```python
from build123d import *

# Parameters (mm, degrees)
SKETCH1_W           = 4.8
SKETCH1_H           = 4.8
BOSS_EXTRUDE1_DEPTH = 20
SKETCH2_W           = 5.2
SKETCH2_H           = 5.2
BOSS_EXTRUDE2_DEPTH = 50
SKETCH3_W           = 17
SKETCH3_H           = 27
BOSS_EXTRUDE3_DEPTH = 10
SKETCH4_W           = 13
SKETCH4_H           = 23
CUT_EXTRUDE1_DEPTH  = 8.5
SKETCH5_W           = 11
SKETCH5_H           = 8.5
CUT_EXTRUDE2_DEPTH  = 8.5
SKETCH6_W           = 5
SKETCH6_H           = 5
BOSS_EXTRUDE4_DEPTH = 81.5
SKETCH7_W           = 5
SKETCH7_H           = 5
BOSS_EXTRUDE5_DEPTH = 43.1
SKETCH9_R           = 0.9
CUT_EXTRUDE4_DEPTH  = 125.748466924
BOSS_EXTRUDE6_DEPTH = 5.2


with BuildPart() as part:
    # Sketch1 → Boss-Extrude1 (new body)
    with BuildSketch(Plane.XY):
        with Locations((2.4, -2.4)):
            Rectangle(SKETCH1_W, SKETCH1_H)
    extrude(amount=BOSS_EXTRUDE1_DEPTH)

    # Sketch2 → Boss-Extrude2 (add)
    with BuildSketch(Plane(origin=(0, 0, 0), x_dir=(-1, 0, 0), z_dir=(0, 0, -1))):
        with Locations((-2.4, -2.4)):
            Rectangle(SKETCH2_W, SKETCH2_H)
    extrude(amount=BOSS_EXTRUDE2_DEPTH)

    # Sketch3 → Boss-Extrude3 (add)
    with BuildSketch(Plane(origin=(0, 0, -50), x_dir=(-1, 0, 0), z_dir=(0, 0, -1))):
        with Locations((-2.4, -2.4)):
            Rectangle(SKETCH3_W, SKETCH3_H)
    extrude(amount=BOSS_EXTRUDE3_DEPTH)

    # Sketch4 → Cut-Extrude1 (cut)
    with BuildSketch(Plane(origin=(0, 0, -60), x_dir=(-1, 0, 0), z_dir=(0, 0, -1))):
        with Locations((-2.4, -2.4)):
            Rectangle(SKETCH4_W, SKETCH4_H)
    extrude(amount=-CUT_EXTRUDE1_DEPTH, mode=Mode.SUBTRACT)

    # Sketch5 → Cut-Extrude2 (cut)
    with BuildSketch(Plane.XZ.offset(15.9)):
        with Locations((2.4, -54.25)):
            Rectangle(SKETCH5_W, SKETCH5_H)
    extrude(amount=-CUT_EXTRUDE2_DEPTH, mode=Mode.SUBTRACT)

    # Sketch6 → Boss-Extrude4 (add)
    with BuildSketch(Plane(origin=(0, 0.2, 0), x_dir=(1, 0, 0), z_dir=(0, 1, 0))):
        with Locations((2.4, 37.5)):
            Rectangle(SKETCH6_W, SKETCH6_H)
    extrude(amount=-BOSS_EXTRUDE4_DEPTH)

    # Sketch7 → Boss-Extrude5 (add)
    with BuildSketch(Plane(origin=(0, 0, -40), x_dir=(-1, 0, 0), z_dir=(0, 0, -1))):
        with Locations((-2.4, -78.8)):
            Rectangle(SKETCH7_W, SKETCH7_H)
    extrude(amount=BOSS_EXTRUDE5_DEPTH)

    # Sketch9 → Cut-Extrude4 (cut, through all)
    with BuildSketch(Plane.XZ.offset(81.3)):
        with Locations((2.4, -80.1)):
            Circle(SKETCH9_R)
    extrude(amount=-CUT_EXTRUDE4_DEPTH, mode=Mode.SUBTRACT)

    # Sketch12 → Boss-Extrude6 (add)
    with BuildSketch(Plane(origin=(5, 0, 0), x_dir=(0, 0, -1), z_dir=(1, 0, 0))):
        Polygon((13.455782968, -5), (35, -40.359932103), (35, -45.359932103), (8.455782968, -5), align=None)
    extrude(amount=-BOSS_EXTRUDE6_DEPTH)


solid = part.part
```
Can you work these out from the model? Positions are in its coordinate system, mm. A direction names the side the tool comes from. Coordinates: 2 decimals unless noted, no trailing zeros. Order: outer loops, then holes, each group sorted by start corner. A loop starts at its lowest first (then second) coordinate and runs counter-clockwise, first axis right, second up.
1. If we section it at B-B (y = -11): Please give me the cut outline in (x, z), then the cut area to 3 significant figures.
2. I'm going to push flat-ended pins straight in: pin 1 (1.5 mm diameter, centred on x = 3, y = -26.5, fed in from +Z); pin 2 (5 mm diameter, centred on x = -0.5, z = -25, fed in from +Y); pin 3 (3 mm diameter, centred on x = 7.5, z = 8.5, fed in from -Y); pin 4 (6 mm diameter, centred on y = -29.5, z = -36.5, fed in from +X). Where does each tip first touch, or does it pass through?
3. If we section it at D-D (z = 2): Please give me the cut outline in (x, y), then the cut area to 3 significant figures.
4. I need wall thicknesses on line 1 (X direction, y = -80.2, z = -80.1); line 2 (Z direction, x = 2.4, y = -79.35); line 3 (Y direction, x = 2.25, z = -61.5). Which ranges of each line are inside material? Lowest first, please.
5. For faces 1 (the face through (-3.1, -15, -52)), 2 (the face through (2, -5, -4)), 3 (the face through (-0.2, -4, -21)), which set-ups out of +Z, -Z, +X, -X, +Y, -Y let a thin tool reach every point of the face, with its end or its side?
6. If we section it at C-C (y = -26): Please give me the cut outline in (x, z).
7. If we section it at A-A (z = -47): Please give me the cut outline in (x, y).
8. Thinking about a two-plate mould opening in Z: for faces 4 (the face through (2, -76.3, -61)), 5 (the face through (2, -5, -31)), 6 (the face through (2.436, -22.432, -24.077)), 7 (the face through (2, -79, -83.1)), which applies, +Z half, -Z half, draft (parallel to the pull), parting line (faces both ways), or undercut?
Entries:
1. outline: (-6.1, -60) - (-4.1, -60) - (-4.1, -51.5) - (-3.1, -51.5) - (-3.1, -50) - (-6.1, -50) - close; (-0.2, -17.11) - (5, -17.11) - (5, -12.4) - (-0.2, -12.4) - close; (-0.1, -40) - (4.9, -40) - (4.9, -35) - (-0.1, -35) - close; (7.9, -51.5) - (8.9, -51.5) - (8.9, -60) - (10.9, -60) - (10.9, -50) - (7.9, -50) - close
1. area: 92.5 mm2
2. pin 1: stops at z = -22.1
2. pin 2: stops at y = 0.2
2. pin 3: passes through
2. pin 4: stops at x = 4.9
3. outline: (0, -4.8) - (4.8, -4.8) - (4.8, 0) - (0, 0) - close
3. area: 23.0 mm2
4. line 1: x = -0.1 to 1.5, 3.3 to 4.9
4. line 2: z = -83.1 to -81, -79.2 to -35
4. line 3: y = -81.3 to -76.3
5. face 1: +Z, -Y
5. face 2: +Z, +X, -X, -Y
5. face 3: +Z, -X, +Y, -Y
6. outline: (-0.2, -26.25) - (5, -26.25) - (5, -22.27) - (-0.2, -22.27) - close; (-0.1, -40) - (4.9, -40) - (4.9, -35) - (-0.1, -35) - close
7. outline: (-0.2, -5) - (5, -5) - (5, 0.2) - (-0.2, 0.2) - close; (-0.1, -81.3) - (4.9, -81.3) - (4.9, -76.3) - (-0.1, -76.3) - close
8. face 4: draft
8. face 5: undercut
8. face 6: undercut
8. face 7: -Z half
